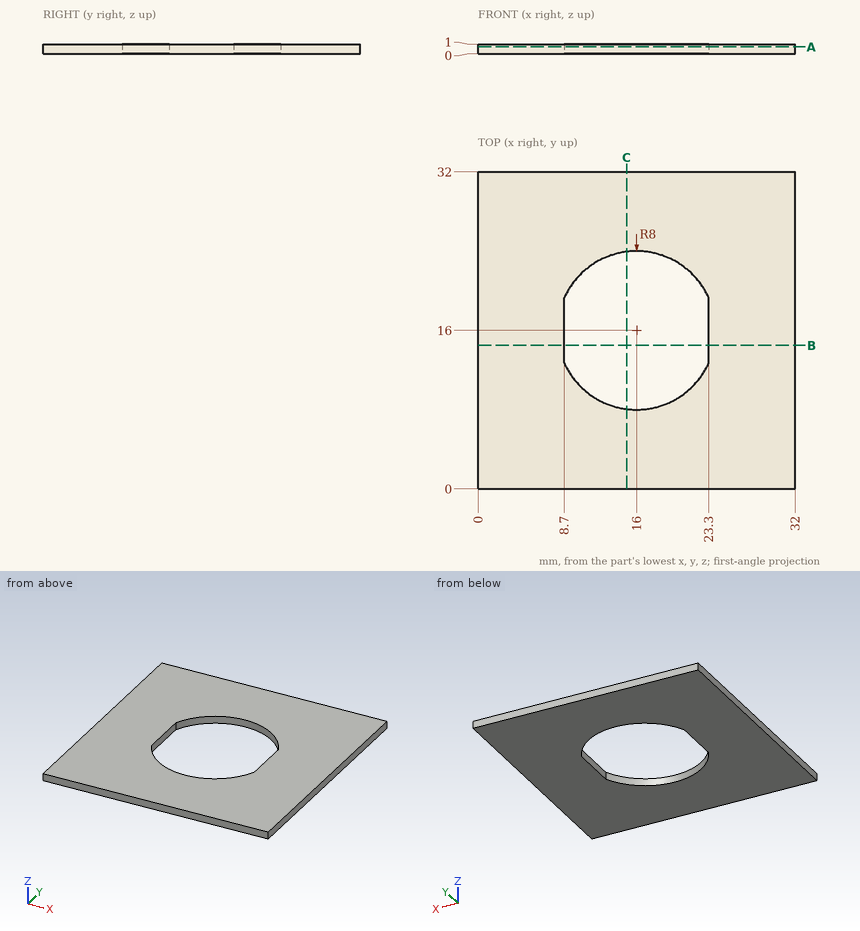
Can you work these out from the drawing? Everything is in mm from the part's minimum corner. Coordinates: 2 decimals unless noted, no trailing zeros. Order: outer loops, then holes, each group sorted by start corner. A loop starts at its lowest first (then second) coordinate and runs counter-clockwise, first axis right, second up. Notation, with made-up numbers: (76, 62) -> (80, 62) arc R31 ccw to (80, 88) -> close; hole circle Ø11 at (57.25, -32.5). An arc over 180 degrees is marked (long way). Return JSON: item names as keys, results as strings.
1) If I drill on probe 1 along X at (y, z) = (13, 0.15); probe 2 along Y at (x, z) = (9.5, 0.85); probe 3 along Y at (x, z) = (10, 0.9), over which ranges is the centre line in solid material (lowest first)?
Conclusion:
{"probe 1": "x = 0 to 8.7, 23.3 to 32", "probe 2": "y = 0 to 11.34, 20.66 to 32", "probe 3": "y = 0 to 10.71, 21.29 to 32"}
2) If we section it at C-C on x = 15: List the corners of the cut face in (y, z) for me.
Conclusion:
{"outline": "(0, 0) -> (8.06, 0) -> (8.06, 1) -> (0, 1) -> close; (23.94, 0) -> (32, 0) -> (32, 1) -> (23.94, 1) -> close"}
3) If we section it at B-B on y = 14.5: List the corners of the cut face in (x, z) for me.
Conclusion:
{"outline": "(0, 0) -> (8.7, 0) -> (8.7, 1) -> (0, 1) -> close; (23.3, 0) -> (32, 0) -> (32, 1) -> (23.3, 1) -> close"}
4) If we section it at A-A on z = 0.7: List the corners of the cut face in (x, y) for me.
Conclusion:
{"outline": "(0, 0) -> (32, 0) -> (32, 32) -> (0, 32) -> close; hole (8.7, 12.73) arc R8 ccw to (23.3, 12.73) -> (23.3, 19.27) arc R8 ccw to (8.7, 19.27) -> close"}
